from build123d import *

# Parameters (mm, degrees)
BOSS_EXTRUDE2_DEPTH = 13.335
SKETCH10_W          = 25.4
SKETCH10_H          = 6.35
CUT_EXTRUDE1_DEPTH  = 14.335
FILLET1_R           = 2.54
FILLET2_R           = 2.032
SKETCH11_R          = 3.81
CUT_EXTRUDE2_DEPTH  = 14.335


with BuildPart() as part:
    # Sketch6 → Boss-Extrude2 (new body)
    with BuildSketch(Plane(origin=(0, 0, 0), x_dir=(1, 0, 0), z_dir=(0, 1, 0))):
        with BuildLine():
            Line((0, 0), (109.1946, 0))
            Line((109.1946, 0), (109.1946, -36.83))
            ThreePointArc((109.1946, -36.83), (54.5973, -59.960965275), (0, -36.83))
            Line((0, -36.83), (0, 0))
        make_face()
    extrude(amount=BOSS_EXTRUDE2_DEPTH)

    # Sketch10 → Cut-Extrude1 (cut, through all)
    with BuildSketch(Plane(origin=(0, 13.335, 0), x_dir=(1, 0, 0), z_dir=(0, 1, 0))):
        with Locations((96.4946, -3.175)):
            Rectangle(SKETCH10_W, SKETCH10_H)
        with Locations((12.7, -3.175)):
            Rectangle(SKETCH10_W, SKETCH10_H)
    extrude(amount=-CUT_EXTRUDE1_DEPTH, mode=Mode.SUBTRACT)

    # Fillet1
    fillet1_edges = [part.edges().sort_by_distance(p)[0] for p in [
        (25.4, 6.6675, 6.35),
        (83.7946, 6.6675, 6.35),
    ]]
    fillet(fillet1_edges, radius=FILLET1_R)

    # Fillet2
    fillet2_edges = [part.edges().sort_by_distance(p)[0] for p in [
        (25.4, 6.6675, 0),
        (83.7946, 6.6675, 0),
    ]]
    fillet(fillet2_edges, radius=FILLET2_R)

    # Sketch11 → Cut-Extrude2 (cut, through all)
    with BuildSketch(Plane.XZ):
        with Locations((54.61, 5.819375203)):
            Circle(SKETCH11_R)
    extrude(amount=-CUT_EXTRUDE2_DEPTH, mode=Mode.SUBTRACT)


solid = part.part
Design review of the part built by this model. Coordinates are the model's own, in mm. A direction names the side the tool comes from. Round coordinates to 2 decimals unless told otherwise and drop trailing zeros. Order: outer loops, then holes, each group sorted by start corner. A loop starts at its lowest first (then second) coordinate and runs counter-clockwise, first axis right, second up.
1) Consider section B-B (y = 6.25). State the section outline as (x, z) points.
The answers:
outline: (0, 6.35) - (22.86, 6.35) arc R2.54 cw to (25.4, 3.81) - (25.4, 2.03) arc R2.03 ccw to (27.43, 0) - (81.76, 0) arc R2.03 ccw to (83.79, 2.03) - (83.79, 3.81) arc R2.54 cw to (86.33, 6.35) - (109.19, 6.35) - (109.19, 36.83) arc R76 ccw to (0, 36.83) - close; hole circle Ø7.62 at (54.61, 5.82)
2) Draft analysis for pull direction X (two halves, no side actions). For faces 1 (the flat face through (98, 7, 6.35)), 2 (the cylindrical face through (83.184, 6.574, 0.579)), 3 (the cylindrical face through (55.45, 6.574, 59.956)), 4 (the cylindrical face through (50.804, 6.574, 5.987)), state which applies: released by +X, released by -X, zero draft, split by the parting line, or undercut.
The answers:
face 1: zero draft
face 2: released by +X
face 3: split by the parting line
face 4: undercut
3) Consider section D-D (z = 53.5). State the section outline as (x, y) points (3 decimals).
The answers:
outline: (23.933, 0) - (85.262, 0) - (85.262, 13.335) - (23.933, 13.335) - close
4) Consider section C-C (x = 100.5). State the section outline as (y, z) points (3 decimals), plus the area to 3 significant figures.
The answers:
outline: (0, 6.35) - (13.335, 6.35) - (13.335, 44.533) - (0, 44.533) - close
area: 509 mm2
5) For L1, parallel to Z at x = 54.61, y = 8; L2, parallel to X at y = 3.25, z = 5.5; L3, parallel to Z at x = 82.5, y = 7.75, list the stretches that pass through material, from the lowest coordinate up.
The answers:
L1: z = 0 to 2.01, 9.63 to 59.96
L2: x = 24.76 to 50.81, 58.41 to 84.44
L3: z = 0.14 to 54.65
6) Machinability: for faces 5 (the flat face through (11, 7, 6.35)), 6 (the flat face through (109.195, 7, 21)), which of the approach directions +Z, -Z, +X, -X, +Y, -Y give a long, thin tool a straight path to every point of the face, cutting with its end or side? Answer none if there is none.
The answers:
face 5: -Z, -X, +Y, -Y
face 6: +Z, -Z, +X, +Y, -Y
7) Consider section A-A (x = 54.61). State the section outline as (y, z) points (3 decimals), plus the area to 3 significant figures.
The answers:
outline: (0, 0) - (13.335, 0) - (13.335, 2.009) - (0, 2.009) - close; (0, 9.629) - (13.335, 9.629) - (13.335, 59.961) - (0, 59.961) - close
area: 698 mm2
8) Clearance check with flat-ended pins moving along their axes: pin 1 Ø4 at (x, y) = (95.5, 8) entering from -Z; pin 2 Ø2 at (y, z) = (4, 2.5) entering from +X; pin 3 Ø1.4 at (y, z) = (7.5, 3) entering from -X. State where each tip first meets the part, or that it passes through.
The answers:
pin 1: stops at z = 6.35
pin 2: stops at x = 83.79
pin 3: stops at x = 25.4
